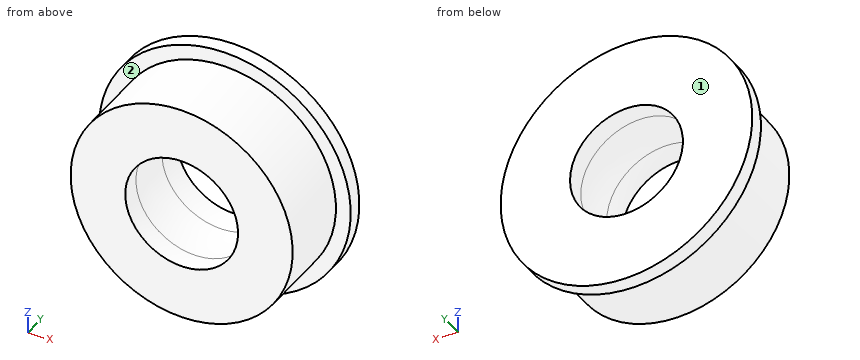
```python
from build123d import *

# Parameters (mm, degrees)
SKETCH1_R           = 6
SKETCH1_R_2         = 3.05
BOSS_EXTRUDE1_DEPTH = 4
SKETCH2_R           = 6.8
SKETCH2_R_2         = 3.05
BOSS_EXTRUDE2_DEPTH = 0.8


with BuildPart() as part:
    # Sketch1 → Boss-Extrude1 (new body)
    with BuildSketch(Plane(origin=(0, 0, 0), x_dir=(1, 0, 0), z_dir=(0, 1, 0))):
        with Locations(Location((0, 0, 0), (0, 0, 270))):
            Circle(SKETCH1_R)
        with Locations(Location((0, 0, 0), (0, 0, 270))):
            Circle(SKETCH1_R_2, mode=Mode.SUBTRACT)
    extrude(amount=BOSS_EXTRUDE1_DEPTH)

    # Sketch2 → Boss-Extrude2 (add)
    with BuildSketch(Plane(origin=(0, 4, 0), x_dir=(1, 0, 0), z_dir=(0, 1, 0))):
        with Locations(Location((0, 0, 0), (0, 0, 270))):
            Circle(SKETCH2_R)
        with Locations(Location((0, 0, 0), (0, 0, 270))):
            Circle(SKETCH2_R_2, mode=Mode.SUBTRACT)
    extrude(amount=BOSS_EXTRUDE2_DEPTH)

    # Sketch3 → Cut-Revolve1 (revolve, cut)
    with BuildSketch(Plane.XY, mode=Mode.PRIVATE) as cut_revolve1_sk:
        with BuildLine():
            Line((-3.05, 0), (-3.05, 4.8))
            ThreePointArc((-3.05, 4.8), (-3.080331229, 4.196956564), (-3.171018764, 3.6))
            ThreePointArc((-3.171018764, 3.6), (-3.292037528, 2.4), (-3.171018764, 1.2))
            ThreePointArc((-3.171018764, 1.2), (-3.080331229, 0.603043436), (-3.05, 0))
        make_face()
    revolve(cut_revolve1_sk.sketch.rotate(Axis((0, 0, 0), (0, 1, 0)), 180), axis=Axis((0, 0, 0), (0, 1, 0)), mode=Mode.SUBTRACT)


solid = part.part
```
Design review of the part built by this model. Coordinates are the model's own, in mm. Face numbers are marked on the shaded views. A direction names the side the tool comes from. Round coordinates to 2 decimals unless told otherwise and drop trailing zeros. Write each loop counter-clockwise with the first axis right and the second up, starting at its lowest first coordinate (ties: lowest second). Pieces come first, ordered by that corner, then holes. Notation, with made-up numbers: (88, 10) -> (123, 10) arc R8 cw to (123, 23) -> close; hole circle Ø6 at (58.25, 74.5). An arc over 180 degrees is marked (long way). Write item = value, one per line. Start each with the question number.
1) Take a section at A-A, the plane x = -3.75. State the section outline as (y, z) points.
2) Tool access review of the marked faces 1 and 2: name each direction out of +Z, -Z, +X, -X, +Y, -Y from which nothing blocks a thin tool from reaching the whole face with its end or side.
3) Wall thickness on probe 1 along Z at (x, y) = (2.75, 4.5); probe 2 along Z at (x, y) = (-1.75, 3.65); probe 3 along X at (y, z) = (2.1, -2): over which ranges is each line inside the solid? List them lowest first. Write a range as from..to.
4) Take a section at B-B, the plane z = 5.75. State the section outline as (x, y) points.
5) Clearance check with a flat-ended pin moving along its axis: pin 1 (2 mm diameter, centred on y = 2, z = 2, fed in from -X). State where the tip first meets the part, or that it passes through.
Results list:
q1.outline = (0, -4.68) -> (4, -4.68) -> (4, -5.67) -> (4.8, -5.67) -> (4.8, 5.67) -> (4, 5.67) -> (4, 4.68) -> (0, 4.68) -> close
q2.face_1 = +Z, -Z, +X, -X, +Y
q2.face_2 = -Y
q3.probe_1 = -6.22..-1.34, 1.34..6.22
q3.probe_2 = -5.74..-2.63, 2.63..5.74
q3.probe_3 = -5.66..-2.61, 2.61..5.66
q4.outline = (-3.63, 4) -> (-1.71, 4) -> (-1.71, 0) -> (1.71, 0) -> (1.71, 4) -> (3.63, 4) -> (3.63, 4.8) -> (-3.63, 4.8) -> close
q5.pin_1 = -5.92
